Build history of the part. All positions in model axes, mm. A direction names the side the tool comes from. Coordinates: 2 decimals unless noted, no trailing zeros. One line per item, written item: value.
```python
from build123d import *

# Parameters (mm, degrees)
BOSS_EXTRUDE1_DEPTH     = 10
SKETCH3_R               = 3
CUT_EXTRUDE1_DEPTH      = 17.173315528
CUT_EXTRUDE1_DEPTH_BACK = 12.173315528
SKETCH4_R               = 3
BOSS_EXTRUDE2_DEPTH     = 17


with BuildPart() as part:
    # Sketch2 → Boss-Extrude1 (new body)
    with BuildSketch(Plane(origin=(707.562217201, 137.847000427, -295.175758868), x_dir=(0.354162423, 0.881836565, -0.311341051), z_dir=(-0.931884805, 0.304841472, -0.196627535))):
        Polygon((-166.545846492, -35.496085413), (-149.545846492, -35.496085413), (-149.545846492, -40.496085413), (-166.545846492, -40.496085413), (-166.545846492, -43.496085413), (-146.545846492, -43.496085413), (-146.545846492, -32.496085413), (-166.545846492, -32.496085413), align=None)
    extrude(amount=BOSS_EXTRUDE1_DEPTH)

    # Sketch3 → Cut-Extrude1 (cut, two sides)
    with BuildSketch(Plane(origin=(18.826454002, -86.301151934, -223.021951761), x_dir=(-0.996915398, -0.028323606, -0.073194688), z_dir=(0.078483686, -0.359772079, -0.92973349))) as cut_extrude1_sk:
        with Locations((-626.324876441, 87.720012572)):
            Circle(SKETCH3_R)
    extrude(amount=CUT_EXTRUDE1_DEPTH, mode=Mode.SUBTRACT)
    extrude(cut_extrude1_sk.sketch, amount=-CUT_EXTRUDE1_DEPTH_BACK, mode=Mode.SUBTRACT)

    # Sketch4 → Boss-Extrude2 (add)
    with BuildSketch(Plane(origin=(112.448325625, 279.987482676, -98.852327665), x_dir=(0.935183927, -0.333959305, 0.117907609), z_dir=(0.354162423, 0.881836565, -0.311341051))):
        with Locations((572.690940182, 195.003128109)):
            Circle(SKETCH4_R)
    extrude(amount=BOSS_EXTRUDE2_DEPTH)


solid = part.part
```
Item 1: Drop flat-ended pins along their axis: P1, Ø8, axis at x = 653.5, y = 12.5, coming from the -Z side; P2, Ø10, axis at y = 13.5, z = -209, coming from the -X side (3 decimals); P3, Ø5, axis at x = 644, y = 8, coming from the -Z side. Give the stop position or say it passes through.
Check result:
P1: stops at z = -217.76
P2: stops at x = 636.025
P3: stops at z = -215.75
Item 2: Probe probe 1 along X at (y, z) = (11.5, -207.25); probe 2 along X at (y, z) = (11.5, -206.25); probe 3 along X at (y, z) = (37, -221). List the from-to ranges inside material, lowest first. Write a range as from..to.
Check result:
probe 1: x = 636.95..641.11, 645.2..647.68
probe 2: x = 636.74..641.51, 644.64..647.47
probe 3: x = 650.46..656.46
Item 3: Tool access for faces 4 (the face through (644.835, 14.311, -214.488)), 5 (the face through (644.527, 16.319, -209.914)), 6 (the face through (640.063, 15.047, -216.514)): list every direction of +Z, -Z, +X, -X, +Y, -Y with a clear straight run to the whole face (end or side of a thin tool).
Check result:
face 4: -X
face 5: none
face 6: -Z, -X, +Y
Item 4: Cut at A-A, the plane x = 641.5. Give the number of separate pieces and of enclosed holes in the cut face, then the cut area to 3 significant figures.
Check result:
separate pieces: 4
enclosed holes: 0
area: 67.7 mm^2
Item 5: Pull direction Z, two halves, no side cores. Call faces 1 (the face through (649.382, 11.999, -214.547)), 2 (the face through (650.34, 22.26, -216.96)), 3 (the face through (654.001, 38.803, -220.544)): released by +Z, released by -Z, zero draft, split by the parting line, or undercut.
Check result:
face 1: released by +Z
face 2: undercut
face 3: released by -Z
